from build123d import *

# Parameters (mm, degrees)
SKETCH1_R            = 84
BOSS_EXTRUDE1_DEPTH  = 10
M6_CLEARANCE_HOLE1_D = 7
SKETCH4_R            = 5
CUT_EXTRUDE1_DEPTH   = 10


with BuildPart() as part:
    # Sketch1 → Boss-Extrude1 (new body)
    with BuildSketch(Plane(origin=(0, 0, 0), x_dir=(1, 0, 0), z_dir=(0, 1, 0))):
        with Locations(Location((0, 0, 0), (0, 0, 270))):
            Circle(SKETCH1_R)
    extrude(amount=BOSS_EXTRUDE1_DEPTH)

    # M6 Clearance Hole1 (through all)
    with Locations(Plane(origin=(0, 10, -76), x_dir=(0, 0, 1), z_dir=(0, 1, 0))):
        with Locations((0, 0), (76, -76), (152, 0), (76, 76)):
            Hole(M6_CLEARANCE_HOLE1_D / 2)

    # Sketch4 → Cut-Extrude1 (cut)
    with BuildSketch(Plane(origin=(0, 10, 0), x_dir=(1, 0, 0), z_dir=(0, 1, 0))):
        with Locations(Location((0, 25, 0), (0, 0, 270))):
            Circle(SKETCH4_R)
        with Locations(Location((25, 0, 0), (0, 0, 270))):
            Circle(SKETCH4_R)
        with Locations(Location((-25, 0, 0), (0, 0, 270))):
            Circle(SKETCH4_R)
        with Locations(Location((0, -25, 0), (0, 0, 270))):
            Circle(SKETCH4_R)
    extrude(amount=-CUT_EXTRUDE1_DEPTH, mode=Mode.SUBTRACT)


solid = part.part
The model under review builds one solid part; all positions refer to its coordinate system, in mm. Round coordinates to 2 decimals unless told otherwise and drop trailing zeros. Order: outer loops, then holes, each group sorted by start corner. A loop starts at its lowest first (then second) coordinate and runs counter-clockwise, first axis right, second up. Notation, with made-up numbers: (-9.75, 71.25) -> (47.25, 71.25) arc R10 cw to (47.25, 76.25) -> close; hole circle Ø11 at (7.25, -20). An arc over 180 degrees is marked (long way). Use CSV: the item, a comma, the result in double quotes. Start each with the question number.
(1) Consider section A-A on z = 0. Write out the cut boundary in (x, y).
(2) Consider section C-C on x = -25. Write out the cut boundary in (y, z), and give its area (3 significant figures).
(3) Consider section B-B on y = 2.75. State how many separate pieces and enclosed holes the cut face has, and give its area (3 significant figures).
(4) Wall thickness on probe 1 along X at (y, z) = (8, 0); probe 2 along X at (y, z) = (6.75, 25); probe 3 along Z at (x, y) = (-28.5, 5.5): over which ranges is each line inside the solid? List them lowest first. Write a range as from..to.
(5) Insertion check: pin 1 (9 mm diameter, centred on x = 0, z = 25, fed in from +Y); pin 2 (2 mm diameter, centred on x = -56.5, y = 2.5, fed in from +Z); pin 3 (5 mm diameter, centred on x = -52.5, y = 7, fed in from -Z); pin 4 (5 mm diameter, centred on x = 47.5, y = 2, fed in from +Z). Each pin has a flat end and moves straight along its axis. Give the tip position at first contact, or say it passes through.
(6) Consider section D-D on z = 25. Write out the cut boundary in (x, y).
(7) Mouldability with a two-part tool opening along Z and no side actions: class faces 1 (the face through (1, 0, -1)), 2 (the face through (0, 5, -30)), 3 (the face through (25.23, 4.93, 80.12)), 4 (the face through (-1.341, 4.93, -79.233)) as pulls with the +Z half, pulls with the -Z half, needs draft (parallel to the pull), parting line crosses it, or undercut.
Responses:
1,outline,"(-84, 0) -> (-79.5, 0) -> (-79.5, 10) -> (-84, 10) -> close; (-72.5, 0) -> (-30, 0) -> (-30, 10) -> (-72.5, 10) -> close; (-20, 0) -> (20, 0) -> (20, 10) -> (-20, 10) -> close; (30, 0) -> (72.5, 0) -> (72.5, 10) -> (30, 10) -> close; (79.5, 0) -> (84, 0) -> (84, 10) -> (79.5, 10) -> close"
2,outline,"(0, -80.19) -> (10, -80.19) -> (10, -5) -> (0, -5) -> close; (0, 5) -> (10, 5) -> (10, 80.19) -> (0, 80.19) -> close"
2,area,"1,500 mm²"
3,separate pieces,"1"
3,enclosed holes,"8"
3,area,"21,700 mm²"
4,probe 1,"-84..-79.5, -72.5..-30, -20..20, 30..72.5, 79.5..84"
4,probe 2,"-80.19..-5, 5..80.19"
4,probe 3,"-79.02..-3.57, 3.57..79.02"
5,pin 1,"through"
5,pin 2,"z = 63.05"
5,pin 3,"z = -67.5"
5,pin 4,"z = 70.93"
6,outline,"(-80.19, 0) -> (-5, 0) -> (-5, 10) -> (-80.19, 10) -> close; (5, 0) -> (80.19, 0) -> (80.19, 10) -> (5, 10) -> close"
7,face 1,"needs draft"
7,face 2,"undercut"
7,face 3,"parting line crosses it"
7,face 4,"undercut"
